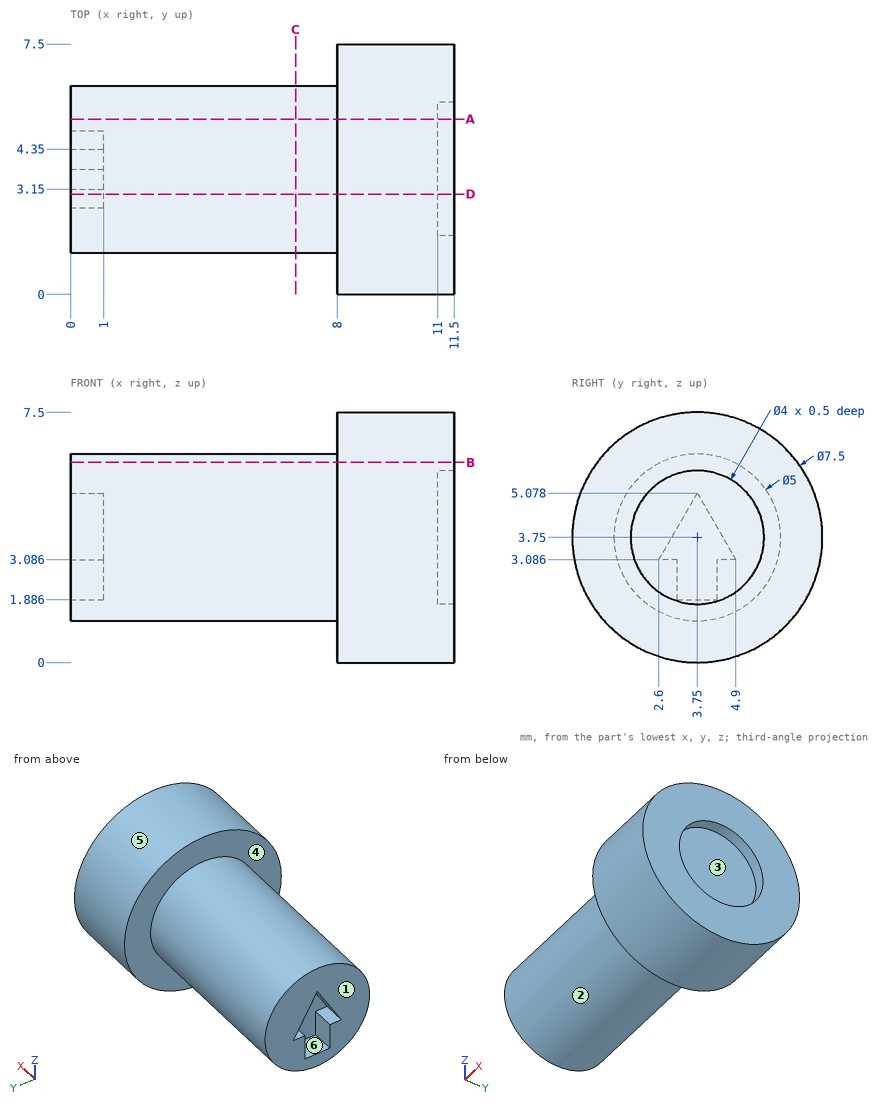
Job drawing, mm, ordinate dimensions from the low corner. One solid piece. A direction names the side the tool comes from. Give positions to 0.01 mm unless a question says otherwise; leave off trailing zeros. Loops run counter-clockwise (first coordinate to the right, second up) from the corner with the lowest first, then second, coordinate; pieces in that order, holes last. Notation, with made-up numbers: (63.5, 74.25) -> (88.5, 74.25) arc R20 cw to (88.5, 106.25) -> close; hole circle Ø5 at (-22, 14.25). An arc over 180 degrees is marked (long way). Use a Markdown table: item, result. Add a question column.
(1) Mould opens along Z. For the marked faces 4, 5 and 6 say: +Z half, -Z half, draft (parallel to the pull), parting line (faces both ways), or undercut.
(2) Slice it at B-B on z = 6. List the corners of the cut face in (x, y).
(3) Slice it at D-D on y = 3. List the corners of the cut face in (x, z) (3 decimals), and give its area (3 significant figures).
(4) Slice it at A-A on y = 5.25. List the corners of the cut face in (x, z).
(5) Drop flat-ended pins along their axis: pin 1 Ø1.5 at (x, y) = (10, 1.5) entering from -Z; pin 2 Ø1.1 at (x, y) = (0.5, 4) entering from +Z; pin 3 Ø3 at (x, z) = (10, 6.5) entering from +Y; pin 4 Ø4.5 at (y, z) = (4.5, 4) entering from +X. Give the stop position or say it passes through.
(6) Slice it at C-C on x = 6.75. List the corners of the cut face in (y, z), and give its area (3 significant figures).
(7) Tool access for the marked faces 1, 2 and 3: list every direction of +Z, -Z, +X, -X, +Y, -Y with a clear straight run to the whole face (end or side of a thin tool).
(8) Wall check: line 1 along Z through (x, y) = (11.3, 3.75); line 2 along X through (y, z) = (2.5, 3.5). Give the ranges that are in metal, low to high.
Filled sheet:
| question | item | result |
|---|---|---|
| 1 | face 4 | draft |
| 1 | face 5 | parting line |
| 1 | face 6 | undercut |
| 2 | outline | (0, 2.66) -> (8, 2.66) -> (8, 0.75) -> (11.5, 0.75) -> (11.5, 6.75) -> (8, 6.75) -> (8, 4.84) -> (0, 4.84) -> close |
| 3 | outline | (0, 1.365) -> (8, 1.365) -> (8, 0.076) -> (11.5, 0.076) -> (11.5, 1.896) -> (11, 1.896) -> (11, 5.604) -> (11.5, 5.604) -> (11.5, 7.424) -> (8, 7.424) -> (8, 6.135) -> (0, 6.135) -> (0, 3.779) -> (1, 3.779) -> (1, 3.086) -> (0, 3.086) -> close |
| 3 | area | 61.3 mm2 |
| 4 | outline | (0, 1.75) -> (8, 1.75) -> (8, 0.31) -> (11.5, 0.31) -> (11.5, 2.43) -> (11, 2.43) -> (11, 5.07) -> (11.5, 5.07) -> (11.5, 7.19) -> (8, 7.19) -> (8, 5.75) -> (0, 5.75) -> close |
| 5 | pin 1 | z = 0.31 |
| 5 | pin 2 | z = 6.25 |
| 5 | pin 3 | y = 7.29 |
| 5 | pin 4 | x = 11.5 |
| 6 | outline | circle Ø5 at (3.75, 3.75) |
| 6 | area | 19.6 mm2 |
| 7 | face 1 | +Z, -Z, -X, +Y, -Y |
| 7 | face 2 | -X |
| 7 | face 3 | +X |
| 8 | line 1 | 0 to 1.75, 5.75 to 7.5 |
| 8 | line 2 | 0 to 11 |
